Autodesk Inventor part; units mm, degrees
ref_plane "YZ Plane" through (0, 0, 0) normal (1, 0, 0) x (0, 1, 0)
ref_plane "XZ Plane" through (0, 0, 0) normal (0, 1, 0) x (-1, 0, 0)
ref_plane "XY Plane" through (0, 0, 0) normal (0, 0, 1) x (1, 0, 0)
sketch "Sketch1" plane through (0, 0, 0) normal (0, 0, 1) x (1, 0, 0)
  line L0 (0, 0) -> (88.9, 0)
  line L1 (88.9, 0) -> (88.9, 44.45)
  line L2 (88.9, 44.45) -> (0, 44.45)
  line L3 (0, 44.45) -> (0, 0)
  line L4 (3.175, 41.275) -> (85.725, 41.275)
  line L5 (85.725, 41.275) -> (85.725, 3.175)
  line L6 (85.725, 3.175) -> (3.175, 3.175)
  line L7 (3.175, 3.175) -> (3.175, 41.275)
  dimension "d0" = 3.175
  dimension "d1" = 88.9
  dimension "d2" = 44.45
extrude "Extrusion1" add sketch "Sketch1" along normal blind 1981.2
hole "Hole1" at (88.9, 22.225, 1958.975) direction (-1, 0, 0) diameter 38.1 end through all
pattern_linear "Rectangular Pattern1" count 2 spacing 889 along (0, 0, -1) of "Hole1"
hole "Hole2" at (88.9, 22.225, 561.975) direction (-1, 0, 0) diameter 38.1 end through all
properties part number "GE-12026-01"
Geometry check sheet. Reference: the model listing, model coordinates, mm. A direction names the side the tool comes from. Give positions to 0.01 mm unless a question says otherwise; leave off trailing zeros. Loops run counter-clockwise (first coordinate to the right, second up) from the corner with the lowest first, then second, coordinate; pieces in that order, holes last.
(1) Section check A-A on z = 1009.5. Record the cut outline in (x, y) (3 decimals).
From the geometry:
outline: (0, 0) - (88.9, 0) - (88.9, 44.45) - (0, 44.45) - close; hole (3.175, 3.175) - (85.725, 3.175) - (85.725, 41.275) - (3.175, 41.275) - close
(2) Set-up check for faces 5 (the flat face through (85.725, 22, 1508)), 6 (the cylindrical face through (87.29, 16.503, 1940.805)): record each of +Z, -Z, +X, -X, +Y, -Y from which the full face is reachable in a straight line by a thin tool's end or side.
From the geometry:
face 5: +Z, -Z
face 6: +X, -X
(3) Section check B-B on x = 17.5. Record the cut outline in (y, z) (3 decimals).
From the geometry:
outline: (0, 0) - (3.175, 0) - (3.175, 1981.2) - (0, 1981.2) - close; (41.275, 0) - (44.45, 0) - (44.45, 1981.2) - (41.275, 1981.2) - close
(4) Depth check by flat-ended pin: pin 1 Ø19 at (y, z) = (13.5, 160) entering from -X; pin 2 Ø23 at (y, z) = (22.225, 1069.975) entering from -X. Enter the tip coordinate at first touch or a pass-through.
From the geometry:
pin 1: stops at x = 0
pin 2: passes through
(5) Thickness scan on L1, parallel to X at y = 19.5, z = 1388.5 (3 decimals); L2, parallel to Y at x = 19.5, z = 1525.5 (3 decimals). Record the ranges inside material, lowest first.
From the geometry:
L1: x = 0 to 3.175, 85.725 to 88.9
L2: y = 0 to 3.175, 41.275 to 44.45
(6) Release check for a two-part mould opening along Y. For faces 1 (the flat face through (45, 44.45, 977)), 2 (the cylindrical face through (87.29, 16.503, 1051.805)), 3 (the flat face through (3.175, 22, 812)), 4 (the flat face through (0, 23, 977)) record: released by +Y, released by -Y, zero draft, split by the parting line, or undercut.
From the geometry:
face 1: released by +Y
face 2: undercut
face 3: undercut
face 4: zero draft
(7) Section check C-C on y = 31. Count the separate pieces of the cut face and the enclosed holes in it, then the cut area to 3 significant figures.
From the geometry:
separate pieces: 8
enclosed holes: 0
area: 11,900 mm2
